Design review of the part shown in the three views and the two pictorial views. Dimensions are in mm from the part's minimum x, y and z. A direction names the side the tool comes from. Give positions to 0.01 mm unless a question says otherwise; leave off trailing zeros. Write each loop counter-clockwise with the first axis right and the second up, starting at its lowest first coordinate (ties: lowest second). Pieces come first, ordered by that corner, then holes. Notation, with made-up numbers: (-22.5, 5) -> (-3.5, 5) arc R12 ccw to (-3.5, 17) -> close; hole circle Ø6 at (-12.5, 24.25). An arc over 180 degrees is marked (long way). Use CSV: the item, a comma, the result in double quotes.
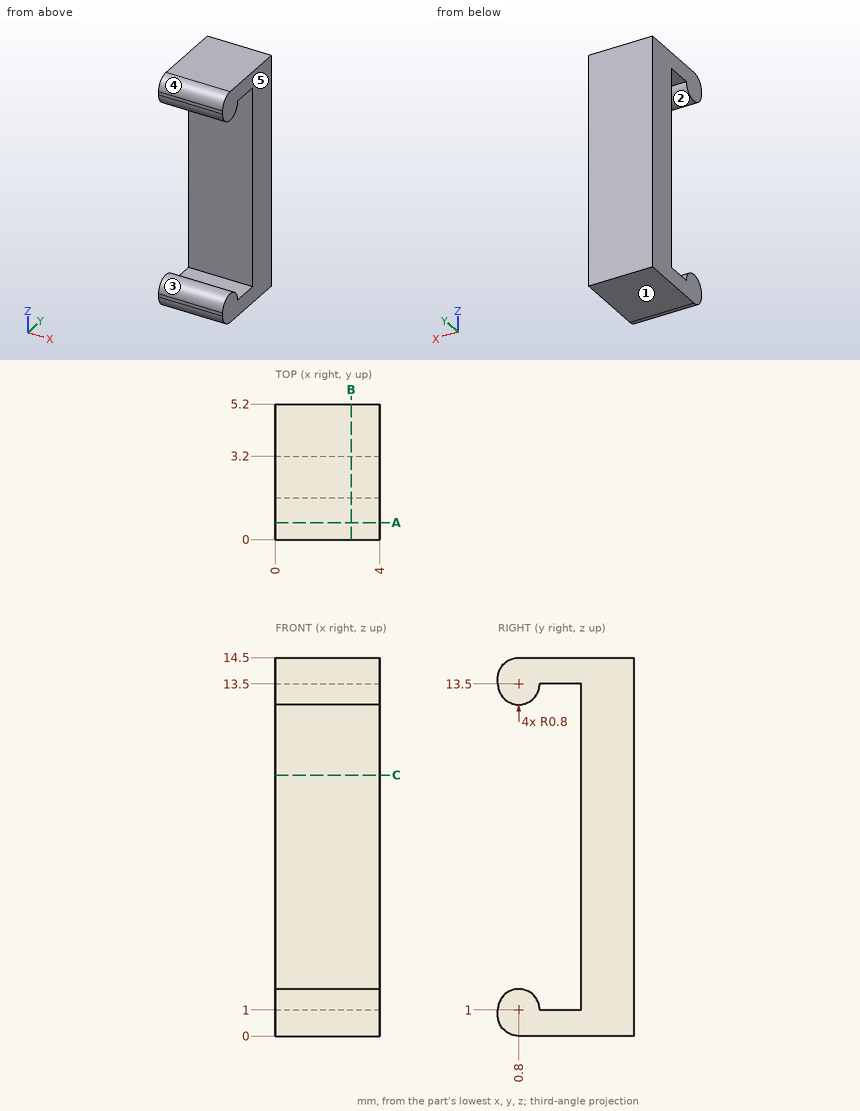
Q1. Consider section C-C (z = 10). Write out the cut boundary in (x, y).
Derived:
outline,"(0, 3.2) -> (4, 3.2) -> (4, 5.2) -> (0, 5.2) -> close"
Q2. Insertion check: pin 1 (1.5 mm diameter, centred on x = 2.5, z = 7.5, fed in from -Y). The pin has a flat end and moves straight along its axis. Give the tip position at first contact, or say it passes through.
Derived:
pin 1,"stops at y = 3.2"
Q3. To check wall thickness, follow probe 1 along Z at (x, y) = (0.6, 1.75); probe 2 along Y at (x, z) = (2.7, 8.5); probe 3 along Z at (x, y) = (2.9, 1.05). State the ranges of each line that lie inside material, in increasing order.
Derived:
probe 1,"z = 0 to 1, 13.5 to 14.5"
probe 2,"y = 3.2 to 5.2"
probe 3,"z = 0 to 1.76, 12.74 to 14.5"
Q4. Consider section B-B (x = 2.9). Write out the cut boundary in (y, z).
Derived:
outline,"(0, 0.8) arc R0.8 ccw to (0.8, 0) -> (5.2, 0) -> (5.2, 14.5) -> (0.8, 14.5) arc R0.8 ccw to (0, 13.7) -> (0, 13.5) arc R0.8 ccw to (1.6, 13.5) -> (3.2, 13.5) -> (3.2, 1) -> (1.6, 1) arc R0.8 ccw to (0, 1) -> close"
Q5. Machinability: for the marked faces 1 and 2, which of the approach directions +Z, -Z, +X, -X, +Y, -Y give a long, thin tool a straight path to every point of the face, cutting with its end or side? Answer none if there is none.
Derived:
face 1,"-Z, +X, -X, +Y, -Y"
face 2,"+X, -X"
Q6. Consider section A-A (y = 0.65). Write out the cut boundary in (x, z), then the cut area to 3 significant figures.
Derived:
outline,"(0, 0.01) -> (4, 0.01) -> (4, 1.79) -> (0, 1.79) -> close; (0, 12.71) -> (4, 12.71) -> (4, 14.49) -> (0, 14.49) -> close"
area,"14.2 mm2"
Q7. The part is to be moulded in two halves that separate along Y. For the marked faces 3, 4 and 5, say which applies: pulls with the +Y half, pulls with the -Y half, needs draft (parallel to the pull), parting line crosses it, or undercut.
Derived:
face 3,"undercut"
face 4,"pulls with the -Y half"
face 5,"needs draft"
